Build history of the part. All positions in model axes, mm. Give positions to 0.01 mm unless a question says otherwise; leave off trailing zeros. Write each loop counter-clockwise with the first axis right and the second up, starting at its lowest first coordinate (ties: lowest second). Pieces come first, ordered by that corner, then holes. Notation, with made-up numbers: (-38.5, 67.25) -> (-2.5, 67.25) arc R23 ccw to (-2.5, 98.25) -> close; hole circle Ø3 at (41, 5.25). An arc over 180 degrees is marked (long way). Put each result on its own line as item: value.
Autodesk Inventor part; units mm, degrees
ref_plane "Work Plane1" through (-22.0572, 0, 0) normal (0, -0.866, -0.5) x (1, 0, 0)
ref_plane "YZ Plane" through (0, 0, 0) normal (1, 0, 0) x (0, 1, 0)
ref_plane "XZ Plane" through (0, 0, 0) normal (0, 1, 0) x (-1, 0, 0)
sketch "Эскиз1" plane through (0, 0, 0) normal (1, 0, 0) x (0, 1, 0)
  line L0 (-12.1244, 0) -> (-6.0622, 10.5)
  line L1 (-6.0622, 10.5) -> (6.0622, 10.5)
  line L2 (6.0622, 10.5) -> (12.1244, 0)
  line L3 (12.1244, 0) -> (6.0622, -10.5)
  line L4 (6.0622, -10.5) -> (-6.0622, -10.5)
  line L5 (-6.0622, -10.5) -> (-12.1244, 0)
  point P0 (0, 0)
  point P1 (0, 0)
  dimension "d0" = 24.2487
extrude "Базовый элемент" add sketch "Эскиз1" along normal blind 12.8
sketch "Эскиз2" plane through (0, 0, 0) normal (0, 0, 1) x (1, 0, 0)
  line L0 (0, 6.0622) -> (0, 12.1244)
  line L1 (0, 12.1244) -> (12.8, 12.1244)
  line L2 (12.8, 6.0622) -> (12.8, 12.1244)
  line L3 (-2.56, 0) -> (15.36, 0)
  line L4 (1.3304, 12.1244) -> (0, 9.82)
  line L5 (11.4696, 12.1244) -> (12.8, 9.82)
  dimension "d3" = 30
  dimension "d4" = 30
  dimension "d5" = 19.64
  dimension "d6" = 19.64
revolve "Фаска1" cut sketch "Эскиз2" angle 360 about axis through (-10, 0, 0) along (1, 0, 0)
sketch "Эскиз3" plane through (12.8, 0, 0) normal (1, 0, 0) x (0, 0, -1)
  arc A0 (-0.625, -1.0825) -> (0.625, -1.0825) centre (0, 0) ccw
hole "Резьба" at (12.8, 0, 0) direction (-1, 0, 0) diameter 12.376 end through all
chamfer "Фаска2" distance 0.8119 angle 30 1 edges at (12.8, 0, 6.188) measured on face at (12.8, 8.4992, -1.032)
chamfer "Фаска3" distance 0.8119 angle 30 1 edges at (0, 0, 6.188) measured on face at (0, 8.4992, -1.032)
ref_plane "Work Plane1" through (-22.0572, 0, 0) normal (0, -0.866, -0.5) x (1, 0, 0)
equation "\"d0\" = 1.1547 * SW"
equation "\"d1\" = KOH"
equation "\"d3\" = ANG1"
equation "\"d4\" = ANG2"
equation "\"d5\" = SW0"
equation "\"d6\" = SW01"
equation "\"d8\" = -0.5 * GD1 + 0.5 * NND"
equation "\"d40\" = -0.5 * GD1 + 0.5 * NND"
equation "\"d10\" = -0.5 * GD1 + 0.5 * NND"
equation "\"d41\" = -0.5 * GD1 + 0.5 * NND"
equation "\"ANG1\" = 30deg"
equation "\"ANG2\" = 30deg"
equation "\"NND\" = 14"
equation "\"KOH\" = 12.8"
equation "\"SW\" = 21"
equation "\"SW0\" = 19.64"
equation "\"SW01\" = SW0"
equation "\"GUL\" = 0.541266 * PTC"
equation "\"LADI\" = 19.64"
equation "\"TOA\" = 30deg"
equation "\"FAWI\" = 30deg"
equation "\"PTC\" = 1.5"
equation "\"THREADDIA\" = 14"
equation "\"E0\" = 1.155 * SW"
equation "\"GAL\" = 0.541266 * PTC"
properties part number "Копия гайки M14x1,5-6H ГОСТ 5915-70" material "Сталь, мягкая"
1) Slice it at A-A (y = 0). Write the cut outline in (x, z).
Filled sheet:
outline: (0, -9.82) -> (0.39, -10.5) -> (12.41, -10.5) -> (12.8, -9.82) -> (12.8, -7) -> (12.33, -6.19) -> (0.47, -6.19) -> (0, -7) -> close; (0, 7) -> (0.47, 6.19) -> (12.33, 6.19) -> (12.8, 7) -> (12.8, 9.82) -> (12.41, 10.5) -> (0.39, 10.5) -> (0, 9.82) -> close
2) Pin check, flat tips, straight feed: pin 1 (1.5 mm diameter, centred on x = 4, z = 4, fed in from -Y); pin 2 (2 mm diameter, centred on x = 3.5, y = 8.5, fed in from +Z); pin 3 (1 mm diameter, centred on x = 2, z = 6, fed in from -Y). Stop position of each tip, or through.
Filled sheet:
pin 1: y = -10.25
pin 2: z = 8.01
pin 3: y = -8.95
3) Pull direction Z, two halves, no side cores. Call faces 1 (the conical face through (0.08, 9.2, -3.82)), 2 (the flat face through (6.316, -9.051, -5.324)), 3 (the cylindrical face through (6.32, 6.04, 1.34)): released by +Z, released by -Z, zero draft, split by the parting line, or undercut.
Filled sheet:
face 1: split by the parting line
face 2: released by -Z
face 3: undercut
4) Wall check: L1, parallel to Z at x = 3.5, y = 0; L2, parallel to Z at x = 12.25, y = -5.5; L3, parallel to Y at x = 6.5, z = -2.25. Give the ranges that are in metal, low to high.
Filled sheet:
L1: -10.5 to -6.19, 6.19 to 10.5
L2: -9.26 to -2.84, 2.84 to 9.26
L3: -10.83 to -5.76, 5.76 to 10.83
5) Slice it at B-B (x = 2.75). Write the cut outline in (y, z), plus the area to 3 significant figures.
Filled sheet:
outline: (-12.12, 0) -> (-6.06, -10.5) -> (6.06, -10.5) -> (12.12, 0) -> (6.06, 10.5) -> (-6.06, 10.5) -> close; hole circle Ø12.38 at (0, 0)
area: 262 mm2
